Geometry: final body of the model. Coordinates: model frame, mm. A direction names the side the tool comes from. Give positions to 0.01 mm unless a question says otherwise; leave off trailing zeros.
Q1. Reachability of faces 1 (the flat face through (4, 3, -15)), 2 (the conical face through (4.61, 5.046, 14.639)) from +Z, -Z, +X, -X, +Y, -Y: full face, straight path, thin tool, end or side. Return the list, or none.
Q2. Line query: line 1 (Z direction, x = -2.5, y = 1.4); line 2 (X direction, y = 4.1, z = -13.5); line 3 (X direction, y = 2.1, z = 10). Output: solid intervals per line, ascending.
Q3. Pin query (flat end, axial travel): pin 1 Ø1 at (x, y) = (15.5, 1.5) entering from -Z; pin 2 Ø0.6 at (y, z) = (4.5, 15.5) entering from -X; pin 3 Ø0.6 at (x, y) = (-15.5, 4) entering from +Z. Return the tip coordinate at first contact, or that it passes through.
from build123d import *

# Parameters (mm, degrees)
SKETCH_1_R                    = 22.5
SKETCH_1_R_2                  = 15
EXTRUDE_1_DEPTH               = 6
PATTERN_LINEAR_45_1_5_1_COUNT = 5
PATTERN_LINEAR_45_1_5_1_PITCH = 1.5
SKETCH_4_W                    = 2
SKETCH_4_H                    = 8
CUT_EXTRUDE_2_DEPTH           = 7
PATTERN_CIRCULAR_1_COUNT      = 4


with BuildPart() as part:
    # Эскиз1 → Вытянуть1 (new body)
    with BuildSketch(Plane(origin=(0, 0, 0), x_dir=(1, 0, 0), z_dir=(0, 1, 0))):
        Circle(SKETCH_1_R)
        Circle(SKETCH_1_R_2, mode=Mode.SUBTRACT)
    extrude(amount=EXTRUDE_1_DEPTH)

    # Эскиз2 → М45х1,5 1й зуб (revolve, cut)
    with BuildSketch(Plane(origin=(0, 0, 0), x_dir=(0, 0, -1), z_dir=(1, 0, 0))):
        Polygon((-21.58, 6), (-22.5, 5.355809065), (-25, 5.355809065), (-25, 6.644190935), (-22.5, 6.644190935), align=None)
    cut_revolve_45_1_5_1 = revolve(axis=Axis((0, 0, 0), (0, 1, 0)), mode=Mode.SUBTRACT)

    # Эскиз3 → Вырез-Повернуть2 (revolve, cut)
    with BuildSketch(Plane(origin=(0, 0, 0), x_dir=(0, 0, -1), z_dir=(1, 0, 0))):
        Polygon((-15, 4.845299462), (-17, 6), (-15, 6), align=None)
    revolve(axis=Axis((0, 0, 0), (0, 1, 0)), mode=Mode.SUBTRACT)

    # М45х1,5 массив1: М45х1,5 1й зуб ×5
    with Locations(*[(0, -i * PATTERN_LINEAR_45_1_5_1_PITCH, 0) for i in range(1, PATTERN_LINEAR_45_1_5_1_COUNT)]):
        add(cut_revolve_45_1_5_1, mode=Mode.SUBTRACT)

    # Эскиз4 → Вытянуть2 (cut, through all)
    with BuildSketch(Plane(origin=(0, 6, 0), x_dir=(1, 0, 0), z_dir=(0, 1, 0))):
        with Locations((15.456832295, 0)):
            Rectangle(SKETCH_4_W, SKETCH_4_H)
    cut_extrude_2 = extrude(amount=-CUT_EXTRUDE_2_DEPTH, mode=Mode.SUBTRACT)

    # Круговой массив1: Вытянуть2 ×4 about axis
    pattern_circular_1_axis = Axis((0, 0, 0), (0, 1, 0))
    for i in range(1, PATTERN_CIRCULAR_1_COUNT):
        add(cut_extrude_2.rotate(pattern_circular_1_axis, i * 360 / PATTERN_CIRCULAR_1_COUNT), mode=Mode.SUBTRACT)


solid = part.part
Computed:
1. face 1: +Y, -Y
1. face 2: +Y
2. line 1: z = -21.58 to -16.46, 16.46 to 21.58
2. line 2: x = -17.56 to -6.54, 6.54 to 17.56
2. line 3: x = -20.09 to -11.18, 11.18 to 20.09
3. pin 1: stops at z = -16.13
3. pin 2: stops at x = -15.69
3. pin 3: stops at z = 16.56
